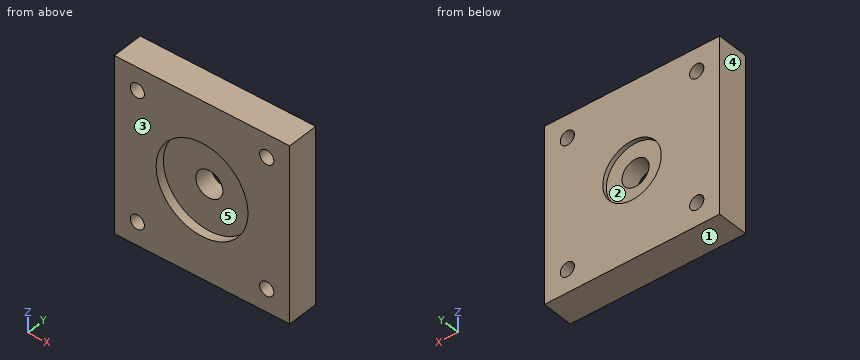
from build123d import *

# Parameters (mm, degrees)
SKETCH1_W           = 42
SKETCH1_H           = 42
SKETCH1_R           = 1.7
BOSS_EXTRUDE1_DEPTH = 7.5
SKETCH2_R           = 11
CUT_EXTRUDE1_DEPTH  = 2.1
SKETCH3_R           = 7
CUT_EXTRUDE2_DEPTH  = 1
SKETCH4_R           = 3.25
CUT_EXTRUDE3_DEPTH  = 10


with BuildPart() as part:
    # Sketch1 → Boss-Extrude1 (new body)
    with BuildSketch(Plane(origin=(0, 0, 0), x_dir=(1, 0, 0), z_dir=(0, 1, 0))):
        Rectangle(SKETCH1_W, SKETCH1_H)
        with Locations((-15.5, 15.5)):
            Circle(SKETCH1_R, mode=Mode.SUBTRACT)
        with Locations((15.5, 15.5)):
            Circle(SKETCH1_R, mode=Mode.SUBTRACT)
        with Locations((15.5, -15.5)):
            Circle(SKETCH1_R, mode=Mode.SUBTRACT)
        with Locations((-15.5, -15.5)):
            Circle(SKETCH1_R, mode=Mode.SUBTRACT)
    extrude(amount=BOSS_EXTRUDE1_DEPTH)

    # Sketch2 → Cut-Extrude1 (cut)
    with BuildSketch(Plane(origin=(0, 0, 0), x_dir=(-1, 0, 0), z_dir=(0, -1, 0))):
        Circle(SKETCH2_R)
    extrude(amount=-CUT_EXTRUDE1_DEPTH, mode=Mode.SUBTRACT)

    # Sketch3 → Cut-Extrude2 (cut)
    with BuildSketch(Plane(origin=(0, 7.5, 0), x_dir=(1, 0, 0), z_dir=(0, 1, 0))):
        Circle(SKETCH3_R)
    extrude(amount=-CUT_EXTRUDE2_DEPTH, mode=Mode.SUBTRACT)

    # Sketch4 → Cut-Extrude3 (cut)
    with BuildSketch(Plane(origin=(0, 6.5, 0), x_dir=(1, 0, 0), z_dir=(0, 1, 0))):
        Circle(SKETCH4_R)
    extrude(amount=-CUT_EXTRUDE3_DEPTH, mode=Mode.SUBTRACT)


solid = part.part
Read the model definition and answer for the solid it produces. Units are mm, in the model's axes. Face numbers are marked on the shaded views. A direction names the side the tool comes from. Round coordinates to 2 decimals unless told otherwise and drop trailing zeros. Write each loop counter-clockwise with the first axis right and the second up, starting at its lowest first coordinate (ties: lowest second). Pieces come first, ordered by that corner, then holes. Notation, with made-up numbers: (-34.5, -23.5) - (22.5, -23.5) arc R23 cw to (22.5, -4.5) - close; hole circle Ø5 at (63.5, -33.75). An arc over 180 degrees is marked (long way). One line per question, with ' | ' between items. Start each with the question number.
1. Find the intervals of material crossed by probe 1 along X at (y, z) = (2.5, -15.5); probe 2 along Z at (x, y) = (14, 3.5), in increasing order. Write a range as [from, to].
2. For a pull along X with two mould halves and no side action, classify the marked faces 3, 4 and 5 as +X half, -X half, draft (parallel to the pull), parting line (faces both ways), or undercut.
3. This flat-tipped pin is pushed along its axis until it touches: pin 1 (4 mm diameter, centred on x = -2, z = 2.5, fed in from +Y). Where does it stop, or does it pass through?
4. Section A-A (y = 3.75) is taken. Determine the outline of the cut face in (x, z).
5. For the marked faces 1 and 2, determine the directions among +Z, -Z, +X, -X, +Y, -Y from which every point of the face is accessible in a straight line to the end or side of a thin tool.
6. Section B-B (z = 0) is taken. Determine the outline of the cut face in (x, y).
7. Section C-C (x = -15.5) is taken. Determine the outline of the cut face in (y, z), and give its area (3 significant figures).
8. Section D-D (z = -15.5) is taken. Determine the outline of the cut face in (x, y), and give its area (3 significant figures).
Filled in:
1) probe 1: [-21, -17.2], [-13.8, 13.8], [17.2, 21] | probe 2: [-21, -16.3], [-14.7, 14.7], [16.3, 21]
2) face 3: draft | face 4: -X half | face 5: undercut
3) pin 1: y = 6.5
4) outline: (-21, -21) - (21, -21) - (21, 21) - (-21, 21) - close; hole circle Ø3.4 at (-15.5, -15.5); hole circle Ø3.4 at (-15.5, 15.5); hole circle Ø6.5 at (0, 0); hole circle Ø3.4 at (15.5, -15.5); hole circle Ø3.4 at (15.5, 15.5)
5) face 1: -Z, +X, -X, +Y, -Y | face 2: +Y
6) outline: (-21, 0) - (-11, 0) - (-11, 2.1) - (-3.25, 2.1) - (-3.25, 6.5) - (-7, 6.5) - (-7, 7.5) - (-21, 7.5) - close; (3.25, 2.1) - (11, 2.1) - (11, 0) - (21, 0) - (21, 7.5) - (7, 7.5) - (7, 6.5) - (3.25, 6.5) - close
7) outline: (0, -21) - (7.5, -21) - (7.5, -17.2) - (0, -17.2) - close; (0, -13.8) - (7.5, -13.8) - (7.5, 13.8) - (0, 13.8) - close; (0, 17.2) - (7.5, 17.2) - (7.5, 21) - (0, 21) - close | area: 264 mm²
8) outline: (-21, 0) - (-17.2, 0) - (-17.2, 7.5) - (-21, 7.5) - close; (-13.8, 0) - (13.8, 0) - (13.8, 7.5) - (-13.8, 7.5) - close; (17.2, 0) - (21, 0) - (21, 7.5) - (17.2, 7.5) - close | area: 264 mm²
